Model file for the job. Use its own axes, mm. Round coordinates to 2 decimals unless told otherwise and drop trailing zeros. Loops run counter-clockwise (first coordinate to the right, second up) from the corner with the lowest first, then second, coordinate; pieces in that order, holes last. Notation, with made-up numbers: M -16,74.5 L 35,74.5 A17 cw 35,96.5 Z; hole C -6.75,64 d10. An arc over 180 degrees is marked long. Use a Markdown table: item, result. Add a question column.
Q1. Probe line 1 (Y direction, x = 5, z = 1.25); line 2 (Z direction, x = 1.75, y = -1.75); line 3 (Z direction, x = -4.75, y = -0.95). List the from-to ranges inside material, lowest first. Write a range as from..to.
Q2. Cut at D-D (z = -3.75). Give the cut face in (x, y), plus the area to 3 significant figures.
Q3. Cut at C-C (z = -1). Give the cut face in (x, y), plus the area to 3 significant figures.
Q4. Cut at B-B (x = 5.5). Give the cut face in (y, z), plus the area to 3 significant figures.
Q5. Cut at A-A (y = 0.85). Give the cut face in (x, z), plus the area to 3 significant figures.
Q6. Pin check, flat tips, straight feed: pin 1 (1.5 mm diameter, centred on x = 3.5, y = -0.5, fed in from -Z); pin 2 (3 mm diameter, centred on x = 0.5, z = 0, fed in from -Y); pin 3 (1.5 mm diameter, centred on x = 2.5, y = 0.5, fed in from +Z); pin 4 (4 mm diameter, centred on x = 0, z = 1.5, fed in from +Y). Stop position of each tip, or through.
from build123d import *

# Parameters (mm, degrees)
F1_DEPTH = 1
F3_DEPTH = 1
F5_DEPTH = 1


with BuildPart() as f1:
    # F0 (on Front) → F1 (new body)
    with BuildSketch(Plane.XZ):
        with BuildLine():
            ThreePointArc((0, 2.5), (1.767767, 1.767767), (2.5, 0))
            ThreePointArc((2.5, 0), (1.767767, -1.767767), (0, -2.5))
            Line((0, -2.5), (0, -4.5))
            ThreePointArc((0, -4.5), (4.5, 0), (0, 4.5))
            Line((0, 4.5), (0, 2.5))
        make_face()
        with BuildLine():
            ThreePointArc((0, -2.5), (-2.5, 0), (0, 2.5))
            Line((0, 2.5), (0, 4.5))
            Line((0, 4.5), (-5.5, 4.5))
            Line((-5.5, 4.5), (-5.5, -4.5))
            Line((-5.5, -4.5), (0, -4.5))
            Line((0, -4.5), (0, -2.5))
        make_face()
    extrude(amount=F1_DEPTH)

    # F2 (on face) → F3 (join)
    with BuildSketch(Plane.XZ.offset(1)):
        with BuildLine():
            Line((0, 2.5), (0, 6.5))
            Line((0, 6.5), (-5.5, 6.5))
            Line((-5.5, 6.5), (-5.5, -6.566851))
            Line((-5.5, -6.566851), (0, -6.566851))
            Line((0, -6.566851), (0, -2.5))
            ThreePointArc((0, -2.5), (-2.5, 0), (0, 2.5))
        make_face()
        with BuildLine():
            ThreePointArc((0, -6.566851), (6.533425, -0.033425), (0, 6.5))
            Line((0, 6.5), (0, 2.5))
            ThreePointArc((0, 2.5), (1.767767, 1.767767), (2.5, 0))
            ThreePointArc((2.5, 0), (1.767767, -1.767767), (0, -2.5))
            Line((0, -2.5), (0, -6.566851))
        make_face()
    extrude(amount=F3_DEPTH)

    # F4 (on face) → F5 (join)
    with BuildSketch(Plane(origin=(0, 0, 0), x_dir=(-1, 0, 0), z_dir=(0, 1, 0))):
        with BuildLine():
            ThreePointArc((0, 2.5), (1.767767, 1.767767), (2.5, 0))
            ThreePointArc((2.5, 0), (1.767767, -1.767767), (0, -2.5))
            Line((0, -2.5), (0, -6.5))
            Line((0, -6.5), (5.5, -6.5))
            Line((5.5, -6.5), (5.5, 6.5))
            Line((5.5, 6.5), (0, 6.5))
            Line((0, 6.5), (0, 2.5))
        make_face()
        with BuildLine():
            ThreePointArc((0, -2.5), (-2.5, 0), (0, 2.5))
            Line((0, 2.5), (0, 6.5))
            ThreePointArc((0, 6.5), (-6.5, 0), (0, -6.5))
            Line((0, -6.5), (0, -2.5))
        make_face()
    extrude(amount=F5_DEPTH)


solid = f1.part
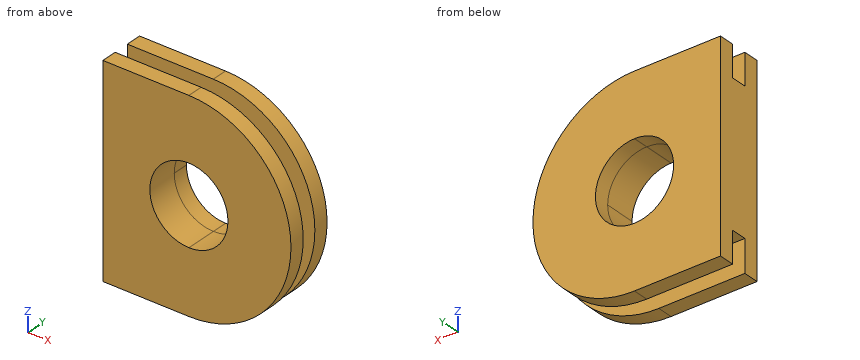
Checked values:
| question | item | result |
|---|---|---|
| 1 | line 1 | y = -2..-1, 0..1 |
| 1 | line 2 | z = -6.33..-1.79, 1.79..6.26 |
| 1 | line 3 | z = -4.5..4.5 |
| 2 | outline | M -5.5,-2 L 5.37,-2 L 5.37,-1 L 2.49,-1 L 2.49,0 L 5.31,0 L 5.31,1 L -5.5,1 Z |
| 2 | area | 29.7 mm^2 |
| 3 | outline | M -5.5,-2 L -2.29,-2 L -2.29,1 L -5.5,1 Z; M 2.29,-2 L 6.46,-2 L 6.46,-1 L 4.39,-1 L 4.39,0 L 6.42,0 L 6.42,1 L 2.29,1 Z |
| 3 | area | 20.0 mm^2 |
| 4 | outline | M -2,-3.56 L -1,-3.56 L -1,3.49 L -2,3.49 Z; M 0,-3.46 L 1,-3.46 L 1,3.46 L 0,3.46 Z |
| 4 | area | 14.0 mm^2 |
| 5 | outline | M -5.5,-6.5 L 0,-6.5 A6.5 ccw 0,6.5 L -5.5,6.5 Z; hole C 0,0 d5 |
| 5 | area | 118 mm^2 |
| 6 | pin 1 | stops at z = -5.87 |
| 6 | pin 2 | passes through |
| 6 | pin 3 | stops at z = 6.26 |
| 6 | pin 4 | stops at y = 1 |
